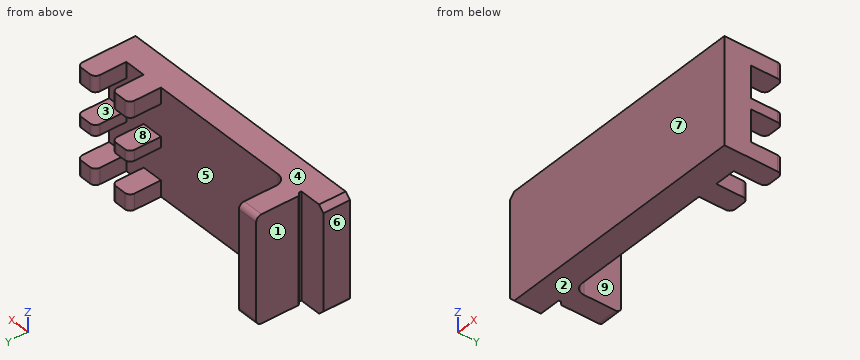
from build123d import *

# Parameters (mm, degrees)
P_IDAT_VYSUNUT_M1_DEPTH  = 10
SKICA2_W                 = 12
SKICA2_H                 = 6
ODEBRAT_VYSUNUT_M1_DEPTH = 6
ZAOBLIT1_R               = 1
ZKOSEN_1_SIZE            = 1
ZAOBLIT2_R               = 2
ODEBRAT_VYSUNUT_M2_DEPTH = 56.192843739


with BuildPart() as part:
    # Skica1 → Přidat vysunutím1 (new, symmetric)
    with BuildSketch(Plane.XY):
        Polygon((-49.5, 0), (0, 0), (0, 11), (-4, 11), (-4, 5), (-8, 5), (-8, 11), (-12, 11), (-12, 5), (-41, 5), (-41, 14), (-45, 14), (-45, 5), (-49.5, 5), align=None)
    extrude(amount=P_IDAT_VYSUNUT_M1_DEPTH, both=True)

    # Skica2 → Odebrat vysunutím1 (cut)
    with BuildSketch(Plane(origin=(0, 11, 0), x_dir=(1, 0, 0), z_dir=(0, 1, 0))):
        with Locations((-6, 4)):
            Rectangle(SKICA2_W, SKICA2_H)
        with Locations((-6, -4)):
            Rectangle(SKICA2_W, SKICA2_H)
    extrude(amount=-ODEBRAT_VYSUNUT_M1_DEPTH, mode=Mode.SUBTRACT)

    # Zaoblit1
    zaoblit1_edges = [part.edges().sort_by_distance(p)[0] for p in [
        (-43, 14, -10),
        (-12, 11, 8.5),
        (-8, 11, 8.5),
        (-4, 11, 8.5),
        (0, 11, 8.5),
        (-8, 11, 0),
        (-8, 11, -8.5),
        (-4, 11, 0),
        (-4, 11, -8.5),
        (-43, 14, 10),
        (0, 11, 0),
        (0, 11, -8.5),
        (-12, 11, 0),
        (-12, 11, -8.5),
    ]]
    fillet(zaoblit1_edges, radius=ZAOBLIT1_R)

    # Zkosení1
    zkosen_1_edges = [part.edges().sort_by_distance(p)[0] for p in [
        (-49.5, 2.5, -10),
        (-49.5, 2.5, 10),
    ]]
    chamfer(zkosen_1_edges, length=ZKOSEN_1_SIZE)

    # Zaoblit2
    zaoblit2_edges = [part.edges().sort_by_distance(p)[0] for p in [
        (-41, 5, 0),
    ]]
    fillet(zaoblit2_edges, radius=ZAOBLIT2_R)

    # Skica3 → Odebrat vysunutím2 (cut, through all)
    with BuildSketch(Plane.XY.offset(10)):
        Polygon((-45, 6), (-44.4, 5.4), (-44.4, 5), (-45, 5), align=None)
    extrude(amount=-ODEBRAT_VYSUNUT_M2_DEPTH, mode=Mode.SUBTRACT)


solid = part.part
For this review, take the finished solid that the model builds, in its own axes (mm). Face numbers are marked on the shaded views. A direction names the side the tool comes from. Give positions to 0.01 mm unless a question says otherwise; leave off trailing zeros. Loops run counter-clockwise (first coordinate to the right, second up) from the corner with the lowest first, then second, coordinate; pieces in that order, holes last.
Item 1: Insertion check: pin 1 (2.5 mm diameter, centred on y = 7.5, z = 8.5, fed in from -X). The pin has a flat end and moves straight along its axis. Give the tip position at first contact, or say it passes through.
Item 2: Tool access review of the marked faces 5, 6, 7, 8 and 9: name each direction out of +Z, -Z, +X, -X, +Y, -Y from which nothing blocks a thin tool from reaching the whole face with its end or side.
Item 3: Take a section at B-B, the plane z = -2. State the section outline as (x, y) points.
Item 4: For line 1 along X through (y, z) = (7, -4.5); line 2 along Y through (x, z) = (-8.5, -3), list the stretches that pass through material, from the lowest coordinate up.
Item 5: Draft analysis for pull direction Z (two halves, no side actions). For the marked faces 1, 2, 3 and 4, state which applies: +Z half, -Z half, draft (parallel to the pull), parting line (faces both ways), or undercut.
Item 6: Take a section at A-A, the plane y = 7.5. State the section outline as (x, z) points, and give its area (3 significant figures).
Item 7: Take a section at C-C, the plane x = -22.5. State the section outline as (y, z) points, and give its area (3 significant figures).
Item 8: Take a section at D-D, the plane y = 11.5. State the section outline as (x, z) points, and give its area (3 significant figures).
Calculated:
1. pin 1: stops at x = -45
2. face 5: +Y
2. face 6: +Z, -Z, -X, +Y, -Y
2. face 7: +Z, -Z, +X, -X, -Y
2. face 8: +X, +Y
2. face 9: +Z, -Z, +Y
3. outline: (-49.5, 0) - (0, 0) - (0, 5) - (-39, 5) arc R2 cw to (-41, 7) - (-41, 14) - (-45, 14) - (-45, 6) - (-44.4, 5.4) - (-44.4, 5) - (-49.5, 5) - close
4. line 1: x = -45 to -41
4. line 2: y = 0 to 5
5. face 1: draft
5. face 2: -Z half
5. face 3: undercut
5. face 4: +Z half
6. outline: (-45, -10) - (-41, -10) - (-41, 10) - (-45, 10) - close; (-12, -10) - (-8, -10) - (-8, -7) - (-12, -7) - close; (-12, -1) - (-8, -1) - (-8, 1) - (-12, 1) - close; (-12, 7) - (-8, 7) - (-8, 10) - (-12, 10) - close; (-4, -10) - (0, -10) - (0, -7) - (-4, -7) - close; (-4, -1) - (0, -1) - (0, 1) - (-4, 1) - close; (-4, 7) - (0, 7) - (0, 10) - (-4, 10) - close
6. area: 144 mm2
7. outline: (0, -10) - (5, -10) - (5, 10) - (0, 10) - close
7. area: 100 mm2
8. outline: (-45, -10) - (-41, -10) - (-41, 10) - (-45, 10) - close
8. area: 80.0 mm2
